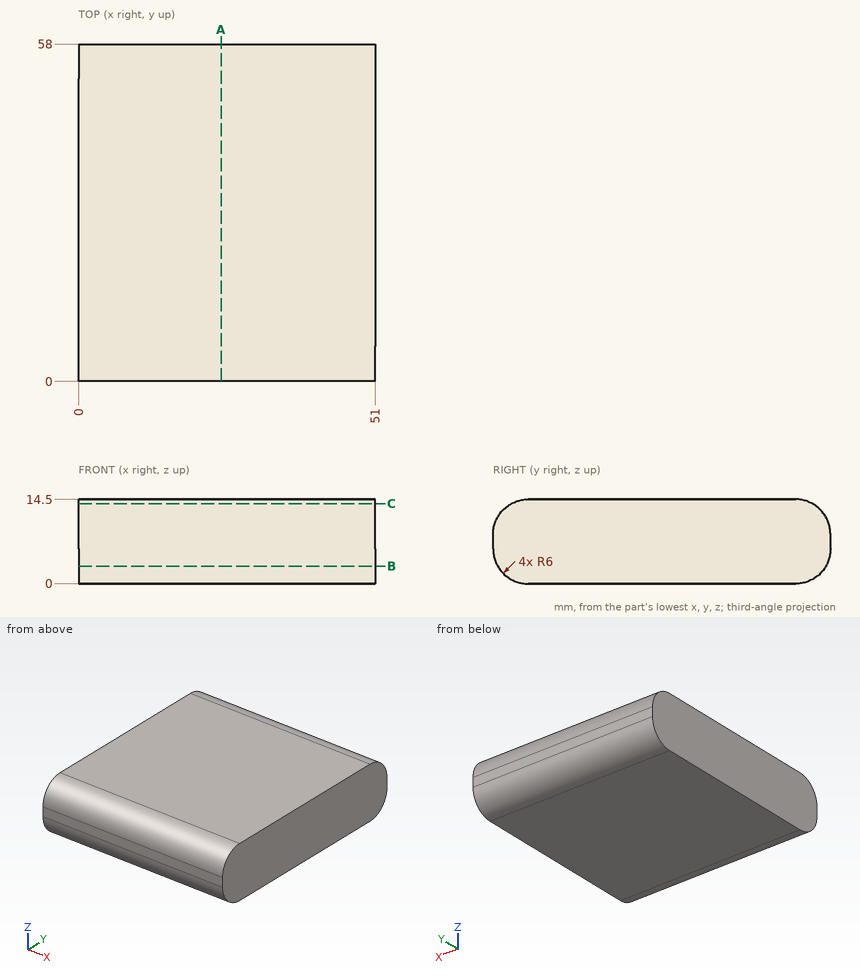
Source: three-view drawing plus pictorial views. Frame: mm from the lowest corner of the part. Coordinates: 2 decimals unless noted, no trailing zeros. Loops run counter-clockwise (first coordinate to the right, second up) from the corner with the lowest first, then second, coordinate; pieces in that order, holes last. Notation, with made-up numbers: (67.25, 81) - (94.25, 81) arc R19 cw to (94.25, 85) - close; hole circle Ø1 at (-4, 54.5). An arc over 180 degrees is marked (long way). One line per item, written item: value. Start each with the question number.
1. Section A-A (x = 24.5). Return the cut outline in (y, z), and give its area (3 significant figures).
2. Section C-C (z = 13.75). Return the cut outline in (x, y).
3. Ray query, L1, parallel to Y at x = 37, z = 2; L2, parallel to Z at x = 18.5, y = 54.5; L3, parallel to Y at x = 10, z = 11.25. Return the intervals inside material, ascending.
4. Contact query for flat-ended pins moving along their axis: P1, Ø4, axis at x = 31, y = 9.5, coming from the -Z side; P2, Ø1.5, axis at x = 28.5, z = 10.5, coming from the +Y side. Output: stop coordinate, or through.
5. Section B-B (z = 3). Return the cut outline in (x, y).
Verdict:
1. outline: (0, 6) arc R6 ccw to (6, 0) - (52, 0) arc R6 ccw to (58, 6) - (58, 8.5) arc R6 ccw to (52, 14.5) - (6, 14.5) arc R6 ccw to (0, 8.5) - close
1. area: 810 mm2
2. outline: (0, 3.1) - (51, 3.1) - (51, 54.9) - (0, 54.9) - close
3. L1: y = 1.53 to 56.47
3. L2: z = 0.55 to 13.95
3. L3: y = 0.67 to 57.33
4. P1: stops at z = 0
4. P2: stops at y = 57.87
5. outline: (0, 0.8) - (51, 0.8) - (51, 57.2) - (0, 57.2) - close
